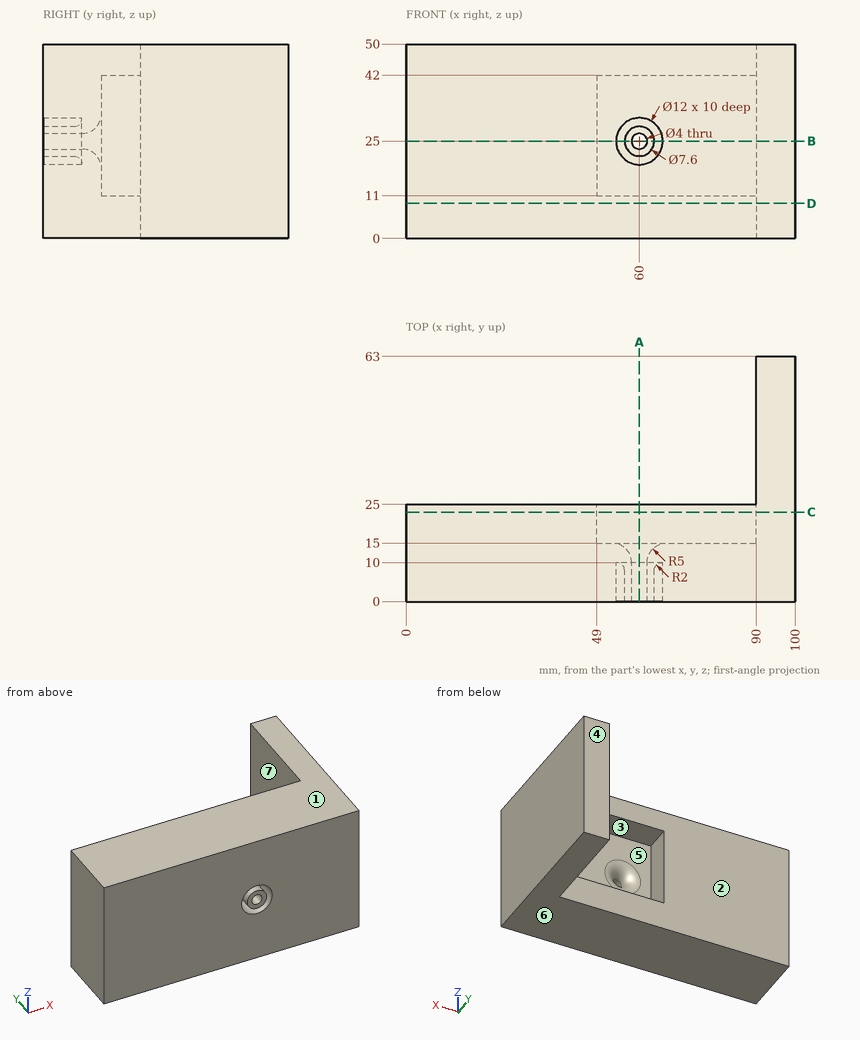
Source: three-view drawing plus pictorial views. Frame: mm from the lowest corner of the part. A direction names the side the tool comes from. Round coordinates to 2 decimals unless told otherwise and drop trailing zeros. Loops run counter-clockwise (first coordinate to the right, second up) from the corner with the lowest first, then second, coordinate; pieces in that order, holes last. Notation, with made-up numbers: M 73.5,-29.75 L 120.5,-29.75 A23 cw 120.5,-1.75 Z; hole C 57,-16 d3. An arc over 180 degrees is marked long. Answer as CSV lines item,"result". Start each with the question number.
(1) Line query: line 1 (X direction, y = 2, z = 25); line 2 (Z direction, x = 60, y = 10.05); line 3 (Z direction, x = 68, y = 20.5). Output: solid intervals per line, ascending. Write a range as [from, to].
(2) Section A-A, the plane x = 60. Output: boundary loops of the cut face in (y, z), plus the area to 3 significant figures.
(3) Reachability of the marked faces 1, 2 and 3 from +Z, -Z, +X, -X, +Y, -Y: full face, straight path, thin tool, end or side. Return the list, or none.
(4) Section C-C, the plane y = 23. Output: boundary loops of the cut face in (x, z).
(5) Draft query along Z for the marked faces 4, 5, 6 and 7. Return one class per face: released by +Z, released by -Z, zero draft, split by the parting line, or undercut.
(6) Section D-D, the plane z = 9. Output: boundary loops of the cut face in (x, y).
(7) Section B-B, the plane z = 25. Output: boundary loops of the cut face in (x, y).
(8) First-contact query: pin 1 (7 mm diameter, centred on x = 60, z = 25, fed in from +Y); pin 2 (15.5 mm diameter, centred on x = 59.5, z = 22, fed in from +Y); pin 3 (5 mm diameter, centred on x = 29, z = 34.5, fed in from +Y). Flat tips, straight axial feed; report the tip coordinate or a pass-through.
Values found:
1,line 1,"x = [0, 54], [56.2, 58], [62, 63.8], [66, 100]"
1,line 2,"z = [0, 23], [27, 50]"
1,line 3,"z = [0, 11], [42, 50]"
2,outline,"M 0,0 L 25,0 L 25,11 L 15,11 L 15,18 A5 ccw 10,23 L 0,23 L 0,21.2 L 8,21.2 A2 cw 10,19.2 L 10,19 L 0,19 Z; M 0,27 L 10,27 A5 ccw 15,32 L 15,42 L 25,42 L 25,50 L 0,50 L 0,31 L 10,31 L 10,30.8 A2 cw 8,28.8 L 0,28.8 Z"
2,area,"827 mm²"
3,face 1,"+Z, +X, -X, +Y, -Y"
3,face 2,"+Z, -Z, -X, +Y"
3,face 3,"+Y"
4,outline,"M 0,0 L 100,0 L 100,50 L 0,50 Z; hole M 49,11 L 90,11 L 90,42 L 49,42 Z"
5,face 4,"zero draft"
5,face 5,"undercut"
5,face 6,"released by -Z"
5,face 7,"undercut"
6,outline,"M 0,0 L 100,0 L 100,63 L 90,63 L 90,25 L 0,25 Z"
7,outline,"M 0,0 L 54,0 L 54,10 L 54.2,10 A2 cw 56.2,8 L 56.2,0 L 58,0 L 58,10 A5 ccw 53,15 L 49,15 L 49,25 L 0,25 Z; M 62,0 L 63.8,0 L 63.8,8 A2 cw 65.8,10 L 66,10 L 66,0 L 100,0 L 100,63 L 90,63 L 90,15 L 67,15 A5 ccw 62,10 Z"
8,pin 1,"stops at y = 13.57"
8,pin 2,"stops at y = 15"
8,pin 3,"stops at y = 25"
